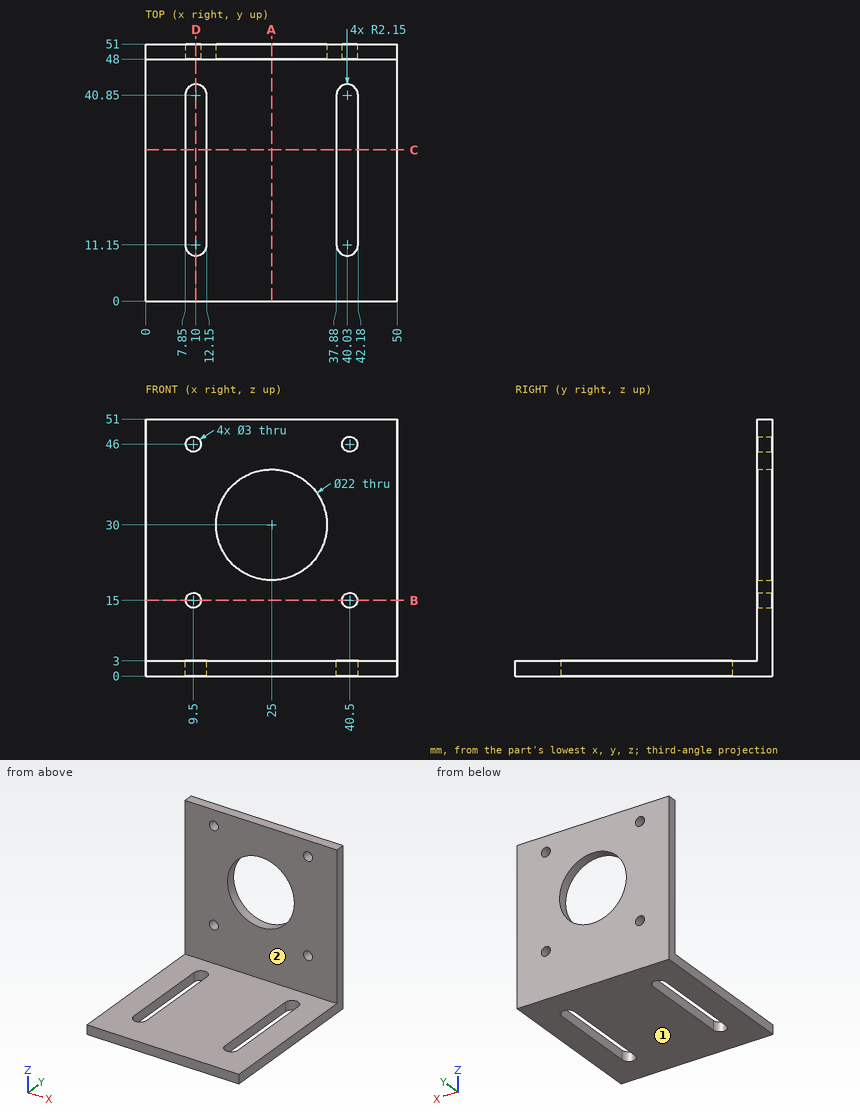
Geometry: see drawing. Coordinates: mm, zero at the bounding-box minimum. A direction names the side the tool comes from. Coordinates: 2 decimals unless noted, no trailing zeros. Loops run counter-clockwise (first coordinate to the right, second up) from the corner with the lowest first, then second, coordinate; pieces in that order, holes last. Notation, with made-up numbers: (81, 11) - (104, 11) arc R26 ccw to (104, 37) - close; hole circle Ø3 at (71, 28.5). An arc over 180 degrees is marked (long way). Answer as CSV lines item,"result".
1. Section B-B (z = 15). Return loops of the section in (x, y), then the cut area to 3 significant figures.
Established:
outline,"(0, 48) - (8, 48) - (8, 51) - (0, 51) - close; (11, 48) - (39, 48) - (39, 51) - (11, 51) - close; (42, 48) - (50, 48) - (50, 51) - (42, 51) - close"
area,"132 mm2"
2. Section A-A (x = 25). Return loops of the section in (y, z).
Established:
outline,"(0, 0) - (51, 0) - (51, 19) - (48, 19) - (48, 3) - (0, 3) - close; (48, 41) - (51, 41) - (51, 51) - (48, 51) - close"
3. Contact query for flat-ended pins moving along their axis: pin 1 (1.5 mm diameter, centred on x = 38, z = 43.5, fed in from -Y); pin 2 (1 mm diameter, centred on x = 14, y = 23.5, fed in from +Z); pin 3 (10 mm diameter, centred on x = 9, y = 35, fed in from -Z); pin 4 (1.8 mm diameter, centred on x = 9.5, z = 46, fed in from +Y). Output: stop coordinate, or through.
Established:
pin 1,"stops at y = 48"
pin 2,"stops at z = 3"
pin 3,"stops at z = 0"
pin 4,"passes through"
4. Ray query, line 1 (X direction, y = 49, z = 15); line 2 (Y direction, x = 22.5, z = 45); line 3 (Z direction, x = 2, y = 20). Return the intervals inside material, ascending.
Established:
line 1,"x = 0 to 8, 11 to 39, 42 to 50"
line 2,"y = 48 to 51"
line 3,"z = 0 to 3"
5. Section C-C (y = 30). Return loops of the section in (x, z).
Established:
outline,"(0, 0) - (7.85, 0) - (7.85, 3) - (0, 3) - close; (12.15, 0) - (37.88, 0) - (37.88, 3) - (12.15, 3) - close; (42.18, 0) - (50, 0) - (50, 3) - (42.18, 3) - close"
6. Reachability of the marked faces 1 and 2 from +Z, -Z, +X, -X, +Y, -Y: full face, straight path, thin tool, end or side. Return the list, or none.
Established:
face 1,"-Z, +X, -X, +Y, -Y"
face 2,"+Z, +X, -X, -Y"
7. Section D-D (x = 10). Return loops of the section in (y, z).
Established:
outline,"(0, 0) - (9, 0) - (9, 3) - (0, 3) - close; (43, 0) - (51, 0) - (51, 13.59) - (48, 13.59) - (48, 3) - (43, 3) - close; (48, 16.41) - (51, 16.41) - (51, 44.59) - (48, 44.59) - close; (48, 47.41) - (51, 47.41) - (51, 51) - (48, 51) - close"
